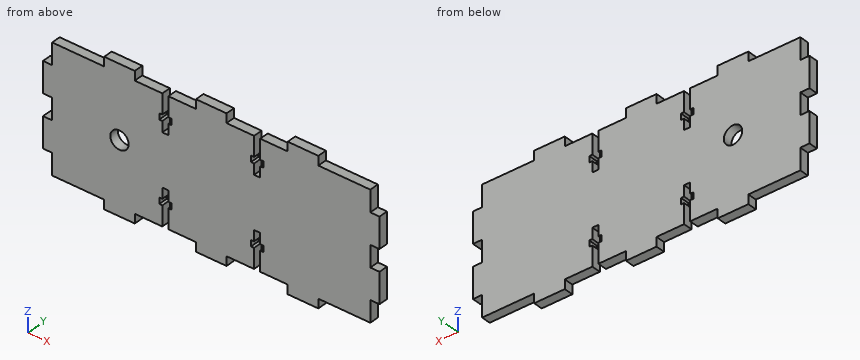
from build123d import *

# Parameters (mm, degrees)
F0_R     = 3
F1_DEPTH = 3


with BuildPart() as f1:
    # F0 (on Front) → F1 (new body)
    with BuildSketch(Plane.XZ):
        Polygon((-47.012073, 8.897897), (-56.012073, 8.897897), (-56.012073, 11.897897), (-66.012073, 11.897897), (-66.012073, 8.897897), (-83.012073, 8.897897), (-83.012073, 1.897897), (-86.012073, 1.897897), (-86.012073, -8.102103), (-83.012073, -8.102103), (-83.012073, -11.602103), (-83.012073, -15.102103), (-86.012073, -15.102103), (-86.012073, -25.102103), (-83.012073, -25.102103), (-83.012073, -32.102103), (-66.012073, -32.102103), (-66.012073, -35.102103), (-56.012073, -35.102103), (-56.012073, -32.102103), (-47.012073, -32.102103), (-47.012073, -25.602103), (-48.012073, -25.602103), (-48.012073, -23.602103), (-47.012073, -23.602103), (-47.012073, -20.102103), (-45.012073, -20.102103), (-45.012073, -23.602103), (-44.012073, -23.602103), (-44.012073, -25.602103), (-45.012073, -25.602103), (-45.012073, -32.102103), (-36.012073, -32.102103), (-36.012073, -35.102103), (-31.012073, -35.102103), (-26.012073, -35.102103), (-26.012073, -32.102103), (-17.012073, -32.102103), (-17.012073, -25.602103), (-18.012073, -25.602103), (-18.012073, -23.602103), (-17.012073, -23.602103), (-17.012073, -20.102103), (-15.012073, -20.102103), (-15.012073, -23.602103), (-14.012073, -23.602103), (-14.012073, -25.602103), (-15.012073, -25.602103), (-15.012073, -32.102103), (-6.012073, -32.102103), (-6.012073, -35.102103), (3.987927, -35.102103), (3.987927, -32.102103), (20.987927, -32.102103), (20.987927, -25.102103), (23.987927, -25.102103), (23.987927, -15.102103), (20.987927, -15.102103), (20.987927, -11.602103), (20.987927, -8.102103), (23.987927, -8.102103), (23.987927, 1.897897), (20.987927, 1.897897), (20.987927, 8.897897), (3.987927, 8.897897), (3.987927, 11.897897), (-6.012073, 11.897897), (-6.012073, 8.897897), (-15.012073, 8.897897), (-15.012073, 2.397897), (-14.012073, 2.397897), (-14.012073, 0.397897), (-15.012073, 0.397897), (-15.012073, -3.102103), (-17.012073, -3.102103), (-17.012073, 0.397897), (-18.012073, 0.397897), (-18.012073, 2.397897), (-17.012073, 2.397897), (-17.012073, 8.897897), (-26.012073, 8.897897), (-26.012073, 11.897897), (-31.012073, 11.897897), (-36.012073, 11.897897), (-36.012073, 8.897897), (-45.012073, 8.897897), (-45.012073, 2.397897), (-44.012073, 2.397897), (-44.012073, 0.397897), (-45.012073, 0.397897), (-45.012073, -3.102103), (-47.012073, -3.102103), (-47.012073, 0.397897), (-48.012073, 0.397897), (-48.012073, 2.397897), (-47.012073, 2.397897), align=None)
        with Locations((-61.012073, -11.602103)):
            Circle(F0_R, mode=Mode.SUBTRACT)
    extrude(amount=F1_DEPTH)


solid = f1.part
Here's how the part is built. I have some questions about the finished solid (model axes, mm). Round coordinates to 2 decimals unless told otherwise and drop trailing zeros. Order: outer loops, then holes, each group sorted by start corner. A loop starts at its lowest first (then second) coordinate and runs counter-clockwise, first axis right, second up. Notation, with made-up numbers: M 80,10 L 89,10 A16 ccw 89,23 Z; hole C 50.5,25 d9. An arc over 180 degrees is marked long. Return JSON: item names as keys, results as strings. Group by question number.
1. If we section it at C-C on x = -16: List the corners of the cut face in (y, z) for me, then the cut area to 3 significant figures.
2. If we section it at B-B on z = -28.5: List the corners of the cut face in (x, y) for me.
3. If we section it at A-A on z = -22: List the corners of the cut face in (x, y) for me.
4. Please list where these lines run through material, in increasing order: probe 1 along X at (y, z) = (-2.6, -22.5); probe 2 along X at (y, z) = (-2.3, 9.5); probe 3 along X at (y, z) = (-0.7, -11.5).
5. I'm going to push flat-ended pins straight in: pin 1 Ø1.5 at (x, y) = (-75, -1.5) entering from -Z; pin 2 Ø1.6 at (x, y) = (-16, -1) entering from +Z; pin 3 Ø0.5 at (x, y) = (-44.5, -1.5) entering from +Z. Where does each tip first touch, or does it pass through?
Reply:
{
 "1": {"outline": "M -3,-20.1 L 0,-20.1 L 0,-3.1 L -3,-3.1 Z", "area": "51.0 mm^2"},
 "2": {"outline": "M -83.01,-3 L -47.01,-3 L -47.01,0 L -83.01,0 Z; M -45.01,-3 L -17.01,-3 L -17.01,0 L -45.01,0 Z; M -15.01,-3 L 20.99,-3 L 20.99,0 L -15.01,0 Z"},
 "3": {"outline": "M -86.01,-3 L -47.01,-3 L -47.01,0 L -86.01,0 Z; M -45.01,-3 L -17.01,-3 L -17.01,0 L -45.01,0 Z; M -15.01,-3 L 23.99,-3 L 23.99,0 L -15.01,0 Z"},
 "4": {"probe 1": "-86.01 to -47.01, -45.01 to -17.01, -15.01 to 23.99", "probe 2": "-66.01 to -56.01, -36.01 to -26.01, -6.01 to 3.99", "probe 3": "-83.01 to -64.01, -58.01 to 20.99"},
 "5": {"pin 1": "z = -32.1", "pin 2": "z = -3.1", "pin 3": "z = 8.9"}
}
